For this review, take the finished solid that the model builds, in its own axes (mm). A direction names the side the tool comes from. Give positions to 0.01 mm unless a question says otherwise; leave off trailing zeros. Loops run counter-clockwise (first coordinate to the right, second up) from the corner with the lowest first, then second, coordinate; pieces in that order, holes last. Notation, with made-up numbers: (72.25, 84) - (98.25, 84) arc R20 cw to (98.25, 102) - close; hole circle Ø11 at (62, 26.25). An arc over 180 degrees is marked (long way). Use CSV: the item, a comma, the result in double quotes. Start each with the question number.
1. For pin 1 (8.5 mm diameter, centred on x = -16.5, z = 19.5, fed in from -Y) (3 decimals); pin 2 (2 mm diameter, centred on y = 8.5, z = 32.5, fed in from -X); pin 3 (19 mm diameter, centred on x = 17, z = 22, fed in from -Y), all flat-tipped, find the tip position at first contact; note any pin that passes through.
2. Wall thickness on line 1 (Y direction, x = 28, z = 8) (3 decimals); line 2 (X direction, y = 28, z = 49); line 3 (X direction, y = 28, z = 44.5): over which ranges is each line inside the solid? List them lowest first.
3. For faces 5 (the flat face through (0, 85, 38.1)), 6 (the cylindrical face through (-16.55, 32.42, 51.66)), 7 (the flat face through (17, 22.225, 18)), list the 3-axis set-ups (+Z, -Z, +X, -X, +Y, -Y) from which the entire face can be reached by the end or side of a thin tool; tool diameter is ignored.
4. Mouldability with a two-part tool opening along Y and no side actions: class faces 1 (the cylindrical face through (61.59, 39.464, 0.133)), 2 (the flat face through (0, 58, 42.875)), 3 (the cylindrical face through (0.4, 45.8, 38.1)), 4 (the flat face through (7.938, -3, 30)) as pulls with the +Y half, pulls with the -Y half, needs draft (parallel to the pull), parting line crosses it, or undercut.
5. Take a section at C-C on y = 98.5. Give the boundary of the cut face in (x, z) (3 decimals), plus the area to 3 significant figures.
6. Take a section at A-A on y = 68. Give the boundary of the cut face in (x, z) (3 decimals).
7. Take a section at B-B on x = -46.5. Give the boundary of the cut face in (y, z) (3 decimals), plus the area to 3 significant figures.
```python
from build123d import *

# Parameters (mm, degrees)
F1_DEPTH = 63.5
F0_W     = 24.6246428497
F0_H     = 19.05
F2_DEPTH = 25.4
F3_DEPTH = 7.9375
F5_R     = 6.35


with BuildPart() as f1:
    # F0 (on Right) → F1 (new body, symmetric)
    with BuildSketch(Plane.YZ):
        Polygon((-41.275, -9.525), (41.275, -9.525), (41.275, 9.525), (22.225, 9.525), (-41.275, 9.525), align=None)
    extrude(amount=F1_DEPTH, both=True)

    # F0 (on Right) → F2 (join, symmetric)
    with BuildSketch(Plane.YZ):
        with BuildLine():
            Line((22.225, 9.525), (41.275, 9.525))
            Line((41.275, 9.525), (41.275, 27.0002))
            ThreePointArc((41.275, 27.0002), (45.9246798487, 38.2255201513), (57.15, 42.8752))
            Line((57.15, 42.8752), (60.325, 42.8752))
            Line((60.325, 42.8752), (60.325, 61.9252))
            Line((60.325, 61.9252), (57.15, 61.9252))
            add(Edge.make_bspline(
                [(56.2913843938, 61.9146440632), (56.5780770871, 61.9191303195), (56.8642886028, 61.9226504349), (57.15, 61.9252)],
                knots=[110.7664159172, 110.7664159172, 110.7664159172, 110.7664159172, 111.5045361635, 111.5045361635, 111.5045361635, 111.5045361635], degree=3))
            ThreePointArc((56.2913843938, 61.9146440632), (32.1525723819, 51.3904488195), (22.225, 27.0002))
            Line((22.225, 27.0002), (22.225, 9.525))
        make_face()
        with Locations((72.6373214248, 52.4002)):
            Rectangle(F0_W, F0_H)
    extrude(amount=F2_DEPTH, both=True)

    # F0 (on Right) → F3 (join, symmetric)
    with BuildSketch(Plane.YZ):
        with BuildLine():
            add(Edge.make_bspline(
                [(-41.275, 9.525), (-40.5899635887, 38.8110076579), (13.2686895658, 61.2414115691), (56.2913843938, 61.9146440632)],
                knots=[0, 0, 0, 0, 110.7664159172, 110.7664159172, 110.7664159172, 110.7664159172], degree=3))
            Line((-41.275, 9.525), (22.225, 9.525))
            Line((22.225, 9.525), (22.225, 27.0002))
            ThreePointArc((22.225, 27.0002), (32.1525723819, 51.3904488195), (56.2913843938, 61.9146440632))
        make_face()
    extrude(amount=F3_DEPTH, both=True)

    # F0 (on Right) → F4 (revolve)
    with BuildSketch(Plane.YZ):
        Polygon((84.9496428497, 61.9252), (84.9496428497, 42.8752), (84.9496428497, 38.1), (111.125, 38.1), (111.125, 66.675), (84.9496428497, 66.675), align=None)
    revolve(axis=Axis((0, 84.9496428497, 52.3875), (0, 0, -1)))

    # F5
    f5_edges = [f1.edges().sort_by_distance(p)[0] for p in [
        (63.5, -41.275, 0),
        (63.5, 41.275, 0),
        (-63.5, 41.275, 0),
        (-63.5, -41.275, 0),
    ]]
    fillet(f5_edges, radius=F5_R)


solid = f1.part
```
Check result:
1,pin 1,"stops at y = 22.225"
1,pin 2,"stops at x = -7.94"
1,pin 3,"stops at y = -39.11"
2,line 1,"y = -41.275 to 41.275"
2,line 2,"x = -7.94 to 7.94"
2,line 3,"x = -25.4 to 25.4"
3,face 5,"-Z, +X, -X, +Y"
3,face 6,"+Z, -X, -Y"
3,face 7,"+Z, +X, -Y"
4,face 1,"pulls with the +Y half"
4,face 2,"undercut"
4,face 3,"undercut"
4,face 4,"needs draft"
5,outline,"(-22.395, 38.1) - (22.395, 38.1) - (22.395, 66.675) - (-22.395, 66.675) - close"
5,area,"1,280 mm²"
6,outline,"(-25.4, 42.875) - (-19.946, 42.875) - (-19.946, 38.1) - (19.946, 38.1) - (19.946, 42.875) - (25.4, 42.875) - (25.4, 61.925) - (19.946, 61.925) - (19.946, 66.675) - (-19.946, 66.675) - (-19.946, 61.925) - (-25.4, 61.925) - close"
7,outline,"(-41.275, -9.525) - (41.275, -9.525) - (41.275, 9.525) - (-41.275, 9.525) - close"
7,area,"1,570 mm²"
